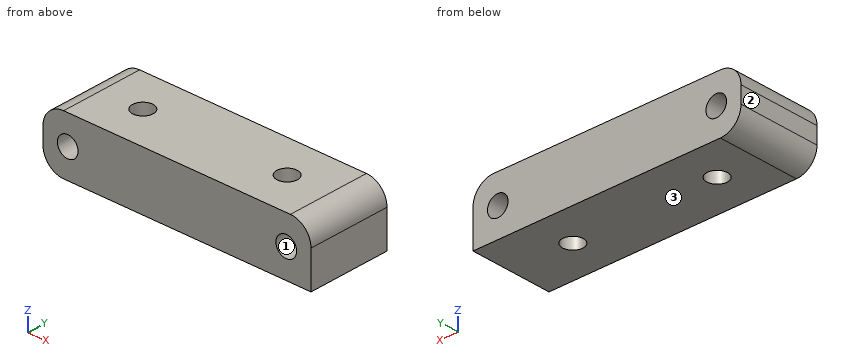
```python
from build123d import *

# Parameters (mm, degrees)
F0_W     = 20
F0_H     = 14
F1_DEPTH = 32.5
F3_D     = 5
F5_D     = 5
F6_R     = 5


with BuildPart() as f1:
    # F0 (on Right) → F1 (new body, symmetric)
    with BuildSketch(Plane.YZ):
        Rectangle(F0_W, F0_H)
    extrude(amount=F1_DEPTH, both=True)

    # F3 (through all)
    with Locations(Plane.XZ.offset(10)):
        with Locations((-26.5, 0), (26.5, 0)):
            Hole(F3_D / 2)

    # F5 (through all)
    with Locations(Plane.XY.offset(7)):
        with Locations((-17.5, 0), (17.5, 0)):
            Hole(F5_D / 2)

    # F6
    f6_edges = [f1.edges().sort_by_distance(p)[0] for p in [
        (32.5, 0, 7),
        (-32.5, 0, -7),
        (-32.5, 0, 7),
    ]]
    fillet(f6_edges, radius=F6_R)


solid = f1.part
```
Source: CAD feature listing. Evaluate the final solid. Frame: model axes, mm. Face numbers are marked on the shaded views. Coordinates: 2 decimals unless noted, no trailing zeros. Write each loop counter-clockwise with the first axis right and the second up, starting at its lowest first coordinate (ties: lowest second). Pieces come first, ordered by that corner, then holes. Notation, with made-up numbers: M 46,58 L 90,58 A20 cw 90,63 Z; hole C 21.5,71 d4. An arc over 180 degrees is marked long. Answer as a JSON object with one key per item and string values.
1. Draft query along X for the marked faces 1, 2 and 3. Return one class per face: released by +X, released by -X, zero draft, split by the parting line, or undercut.
Evaluation:
{"face 1": "undercut", "face 2": "released by -X", "face 3": "zero draft"}
2. Cut plane A-A on z = 0. Output: boundary loops of the cut face in (x, y), plus the area to 3 significant figures.
Evaluation:
{"outline": "M -32.5,-10 L -29,-10 L -29,10 L -32.5,10 Z; M -24,-10 L 24,-10 L 24,10 L -24,10 Z; M 29,-10 L 32.5,-10 L 32.5,10 L 29,10 Z; hole C -17.5,0 d5; hole C 17.5,0 d5", "area": "1,060 mm^2"}
3. Ray query, L1, parallel to X at y = 6.5, z = 0.25; L2, parallel to Y at x = 17.5, z = 3.75; L3, parallel to Z at x = 26.5, y = 3.25. Return the intervals inside material, ascending.
Evaluation:
{"L1": "-32.5 to -28.99, -24.01 to 24.01, 28.99 to 32.5", "L2": "-10 to -2.5, 2.5 to 10", "L3": "-7 to -2.5, 2.5 to 7"}
4. Cut plane D-D on x = -26.5. Output: boundary loops of the cut face in (y, z).
Evaluation:
{"outline": "M -10,-7 L 10,-7 L 10,-2.5 L -10,-2.5 Z; M -10,2.5 L 10,2.5 L 10,7 L -10,7 Z"}
5. Cut plane C-C on x = -16. Output: boundary loops of the cut face in (y, z).
Evaluation:
{"outline": "M -10,-7 L -2,-7 L -2,7 L -10,7 Z; M 2,-7 L 10,-7 L 10,7 L 2,7 Z"}
6. Cut plane B-B on y = -1.5. Output: boundary loops of the cut face in (x, z).
Evaluation:
{"outline": "M -32.5,-2 A5 ccw -27.5,-7 L -19.5,-7 L -19.5,7 L -27.5,7 A5 ccw -32.5,2 Z; M -15.5,-7 L 15.5,-7 L 15.5,7 L -15.5,7 Z; M 19.5,-7 L 32.5,-7 L 32.5,2 A5 ccw 27.5,7 L 19.5,7 Z; hole C -26.5,0 d5; hole C 26.5,0 d5"}
